Autodesk Inventor part; units mm, degrees
ref_plane "YZ Plane" through (0, 0, 0) normal (1, 0, 0) x (0, 1, 0)
ref_plane "XZ Plane" through (0, 0, 0) normal (0, 1, 0) x (-1, 0, 0)
ref_plane "XY Plane" through (0, 0, 0) normal (0, 0, 1) x (1, 0, 0)
sketch "Sketch1" plane through (0, 0, 0) normal (0, 1, 0) x (-1, 0, 0)
  line L0 (0, 0) -> (38.1, -25.4)
  line L1 (38.1, -25.4) -> (0, -25.4)
  line L2 (0, -25.4) -> (0, -57.5469)
  line L3 (0, -57.5469) -> (-28.575, -25.4)
  line L4 (-28.575, -25.4) -> (0, 0)
  dimension "d0" = 38.1
  dimension "d2" = 25.4
  dimension "d3" = 28.575
extrude "Extrusion1" add sketch "Sketch1" along normal blind 25.4
sketch "Sketch2" plane through (0, 25.4, 0) normal (0, 1, 0) x (1, 0, 0)
  line L0 (-38.1, 25.4) -> (0, 0)
  line L1 (-11.9592, 7.9728) -> (19.3376, 35.7921)
  line L2 (0, 0) -> (28.575, 25.4)
  line L3 (28.575, 25.4) -> (0, 57.5469)
  point P0 (0, 25.4)
  dimension "d6" = 5.08
extrude "Extrusion2" cut sketch "Sketch2" against normal blind 49.2125
sketch "Sketch3" plane through (19.3376, 0, -35.7921) normal (0.6643638, 0, 0.7474093) x (0.7474093, 0, -0.6643638)
  line L0 (-32.3668, 19.05) -> (-9.5068, 19.05)
  line L1 (-9.5068, 19.05) -> (-9.5068, 6.35)
  line L2 (-9.5068, 6.35) -> (-32.3668, 6.35)
  line L3 (-32.3668, 6.35) -> (-32.3668, 19.05)
  line L4 (0, 25.4) -> (0, 0)
  line L5 (-41.8736, 25.4) -> (0, 25.4)
  point P0 (-38.2321, 0)
  point P1 (-9.5068, 12.7)
  point P2 (0, 12.7)
  point P3 (-20.9368, 19.05)
  point P4 (-20.9368, 25.4)
  dimension "d9" = 12.7
  dimension "d10" = 22.86
extrude "Extrusion3" cut sketch "Sketch3" against normal blind 82.55
sketch "Sketch4" plane through (19.3376, 0, -35.7921) normal (0.6643638, 0, 0.7474093) x (0.7474093, 0, -0.6643638)
  point P0 (-38.2321, 0)
sketch "Sketch5" plane through (19.3376, 0, -35.7921) normal (0.6643638, 0, 0.7474093) x (0.7474093, 0, -0.6643638)
  line L0 (-9.5068, 6.35) -> (-9.5068, 19.05)
  line L1 (-9.5068, 15.24) -> (-6.9668, 15.24)
  line L2 (-6.9668, 15.24) -> (-6.9668, 10.16)
  line L3 (-6.9668, 10.16) -> (-9.5068, 10.16)
  line L4 (-9.5068, 10.16) -> (-9.5068, 15.24)
  point P0 (-38.2321, 0)
  point P1 (-6.9668, 12.7)
  point P2 (-9.5068, 12.7)
  dimension "d13" = 2.54
  dimension "d14" = 5.08
extrude "Extrusion4" cut sketch "Sketch5" against normal blind 36.5125
sketch "Sketch7" plane through (0, 0, -25.4) normal (0, 0, -1) x (-1, 0, 0)
  line L0 (0, 25.4) -> (38.1, 25.4)
  line L1 (38.1, 0) -> (38.1, 31.4433)
  line L2 (38.1, 31.4433) -> (13.5942, 73.8886)
  line L3 (0, 66.04) -> (0, 19.05)
  line L4 (13.5942, 73.8886) -> (0, 66.04)
  point P0 (0, 0)
extrude "Extrusion6" add sketch "Sketch7" against normal blind 20.6375
sketch "Sketch8" plane through (-38.1, 25.4, -4.7625) normal (0, -1, 0) x (1, 0, 0)
  line L0 (0, -20.6375) -> (26.1408, -3.2103)
  line L1 (26.1408, -3.2103) -> (38.1, -13.8407)
  line L2 (38.1, -13.8407) -> (38.1, 0)
  line L3 (0, 0) -> (38.1, 0)
  line L4 (0, -20.6375) -> (0, 0)
  point P0 (38.1, 4.7625)
extrude "Extrusion7" cut sketch "Sketch8" against normal blind 74.6125
sketch "Sketch9" plane through (0, 25.4, -25.4) normal (1, 0, 0) x (0, 0, -1)
  line L0 (0, 0) -> (-6.7968, 0)
  line L1 (-17.4272, -25.4) -> (-17.4272, 47.5446)
  line L2 (0, 0) -> (-17.4272, 0)
  line L3 (-17.4272, 0) -> (0, 48.4886)
  line L4 (0, 48.4886) -> (-17.4272, 48.4886)
  line L5 (-17.4272, 48.4886) -> (-17.4272, 0)
  point P0 (-25.4, -25.4)
extrude "Extrusion8" cut sketch "Sketch9" against normal blind 92.075
sketch "Sketch10" plane through (0, 25.4, 0) normal (0, 1, 0) x (1, 0, 0)
  line L0 (0, 25.4) -> (0, 18.6032)
  line L1 (0, 18.6032) -> (19.3376, 35.7921)
  line L2 (19.3376, 35.7921) -> (0, 57.5469)
  line L3 (0, 57.5469) -> (0, 25.4)
  line L4 (5.08, 51.054) -> (5.08, 24.93)
  line L5 (5.08, 24.93) -> (5.08, 23.1187)
  line L6 (5.08, 52.3795) -> (5.08, 51.054)
  point P0 (0, 0)
extrude "Extrusion9" add sketch "Sketch10" along normal blind 25.4
ref_plane "Work Plane1" through (0, -6.35, -128.016) normal (0, 0, -1) x (0, 1, 0)
sketch "Sketch11" plane through (0, -6.35, -128.016) normal (0, 0, -1) x (0, 1, 0)
  line L0 (57.15, 19.3376) -> (57.15, 0)
  line L1 (57.15, 0) -> (31.75, 19.3376)
  line L2 (57.15, 19.3376) -> (6.35, 19.3376)
  line L3 (31.75, 19.3376) -> (57.15, 19.3376)
  line L4 (57.15, 19.3376) -> (57.15, 0)
  point P0 (6.35, 0)
  dimension "d27" = 25.4
extrude "Extrusion10" cut sketch "Sketch11" against normal blind 209.55
sketch "Sketch12" plane through (0, 0, -57.5469) normal (-1, 0, 0) x (0, 0, 1)
  circle A0 centre (19.3199, 35.56) radius 1.778
  line L0 (6.4929, 66.04) -> (6.4929, 0)
  line L1 (0, 50.8) -> (32.1469, 50.8)
  point P0 (57.5469, 0)
  dimension "d30" = 3.556
  dimension "d31" = 12.827
  dimension "d32" = 15.24
extrude "Extrusion11" cut sketch "Sketch12" against normal blind 209.55
ref_plane "Work Plane2" through (2.54, 0, -57.5469) normal (-1, 0, 0) x (0, 0, 1)
sketch "Sketch13" plane through (2.54, 0, -57.5469) normal (-1, 0, 0) x (0, 0, 1)
  circle A0 centre (19.3199, 35.56) radius 1.778
  circle A1 centre (19.3199, 35.56) radius 3.81
  point P0 (57.5469, 0)
  dimension "d36" = 7.62
extrude "Extrusion12" cut sketch "Sketch13" against normal blind 209.55 contours A0 | A1
sketch "Sketch14" plane through (0, 0, -25.4) normal (0, 0, -1) x (-1, 0, 0)
  circle A0 centre (25.4, 25.4) radius 1.778
  line L0 (38.1, 0) -> (38.1, 31.4433)
  line L1 (0, 0) -> (38.1, 0)
  dimension "d39" = 3.556
  dimension "d40" = 12.7
  dimension "d41" = 25.4
extrude "Extrusion13" cut sketch "Sketch14" against normal blind 115.8875
ref_plane "Work Plane3" through (0, 0, -22.86) normal (0, 0, -1) x (-1, 0, 0)
sketch "Sketch15" plane through (0, 0, -22.86) normal (0, 0, -1) x (-1, 0, 0)
  circle A0 centre (25.4, 25.4) radius 1.778
  circle A1 centre (25.4, 25.4) radius 3.81
  point P0 (0, 0)
  dimension "d45" = 7.62
extrude "Extrusion14" cut sketch "Sketch15" against normal blind 115.8875
sketch "Sketch16" plane through (0, 0, 0) normal (0, -1, 0) x (1, 0, 0)
  circle A0 centre (-11.9592, -15.5928) radius 1.778
  point P0 (0, 0)
extrude "Extrusion15" cut sketch "Sketch16" against normal blind 15.24
sketch "Sketch17" plane through (-11.9592, 0, -7.9728) normal (0.6643638, 0, 0.7474093) x (0.7474093, 0, -0.6643638)
  circle A0 centre (6.9668, 12.8573) radius 0.889
  circle A1 centre (34.9068, 12.8573) radius 0.889
  line L0 (32.3668, 6.35) -> (9.5068, 6.35)
  point P0 (3.6416, 0)
  point P1 (20.9368, 6.35)
  dimension "d50" = 27.94
  dimension "d51" = 1.778
  dimension "d52" = 1.778
  dimension "d53" = 13.97
extrude "Extrusion16" cut sketch "Sketch17" against normal blind 3.81 contours A0
sketch "Sketch19" plane through (0, 0, 0) normal (0, -1, 0) x (1, 0, 0)
  line L0 (-16.51, -25.4) -> (-14.7303, -25.4)
  line L1 (-16.51, -25.4) -> (-23.1531, -15.4354)
  line L2 (-29.21, -19.4733) -> (-21.59, -14.3933)
  line L3 (-11.43, -25.4) -> (-17.5429, -11.6953)
  line L4 (-11.9592, -7.9728) -> (-26.2667, -17.5112)
  line L5 (0, -25.4) -> (-38.1, -25.4)
  point P0 (0, 0)
extrude "Extrusion18" cut sketch "Sketch19" against normal blind 7.62
chamfer "Chamfer1" distance 1.5875 angle 45 1 edges at (-17.5429, 3.81, -11.6953)
properties part number "Thumb Base2"
Geometry check sheet. Reference: the model listing, model coordinates, mm. A direction names the side the tool comes from. Round coordinates to 2 decimals unless told otherwise and drop trailing zeros. Write each loop counter-clockwise with the first axis right and the second up, starting at its lowest first coordinate (ties: lowest second). Pieces come first, ordered by that corner, then holes.
Item 1: Material ranges on line 1 along Y through (x, z) = (-25.4, -19.75); line 2 along Y through (x, z) = (-27.5, -19); line 3 along Z through (x, y) = (6, 35.56), recorded low to high.
Determined:
line 1: y = 0 to 21.59, 29.21 to 53.44
line 2: y = 0 to 22.22, 28.58 to 49.8
line 3: z = -50.8 to -42.04, -34.42 to -23.94
Item 2: Section check C-C (z = -48). Record the boundary of the cut face in (x, y).
Determined:
outline: (0, 0) - (8.49, 0) - (8.49, 39.65) - (0, 50.8) - close
Item 3: Access from +Z, -Z, +X, -X, +Y, -Y to the whole of each face (thin tool, end or side, straight path). Record for faces 5 (the face through (-21.594, 25.568, -19.613)), 6 (the face through (0, 57, -23)), 7 (the face through (-12, 15.24, -16)), 8 (the face through (7.164, 12.736, -39.001)).
Determined:
face 5: +Z
face 6: +Z, -Z, +X, +Y
face 7: -Y
face 8: +Z, -X
Item 4: Section check D-D (y = 65). Record the boundary of the cut face in (x, z), plus the area to 3 significant figures.
Determined:
outline: (-18.73, -25.4) - (0, -25.4) - (0, -22.21) - (-18.73, -22.21) - close
area: 59.8 mm2
Item 5: Go/stop test with flat-tipped pins: pin 1 Ø12 at (y, z) = (35.56, -38.227) entering from -X; pin 2 Ø3 at (x, z) = (-17.5, -16) entering from -Y; pin 3 Ø3 at (x, y) = (-7, 3.5) entering from -Z; pin 4 Ø13.5 at (x, z) = (-2, -25.5) entering from -Y. Record where each tip stops, or that it passes through.
Determined:
pin 1: stops at x = 0
pin 2: stops at y = 7.62
pin 3: stops at z = -25.4
pin 4: stops at y = 0
Item 6: Mould release check, pull along X, two halves, no side actions. Record for faces 1 (the face through (-24.847, 19.835, -16.564)), 2 (the face through (-24, 24, -22.86)), 3 (the face through (-9.723, 12.611, -19.767)), 4 (the face through (-18, 7.62, -18)): +X half, -X half, draft (parallel to the pull), parting line (faces both ways), or undercut.
Determined:
face 1: -X half
face 2: undercut
face 3: +X half
face 4: undercut
Item 7: Section check B-B (x = -25.4). Record the boundary of the cut face in (y, z), plus the area to 3 significant figures.
Determined:
outline: (0, -25.4) - (23.62, -25.4) - (23.62, -22.86) - (21.59, -22.86) - (21.59, -16.93) - (0, -16.93) - close; (27.18, -25.4) - (53.44, -25.4) - (53.44, -18.05) - (50.33, -16.93) - (29.21, -16.93) - (29.21, -22.86) - (27.18, -22.86) - close
area: 397 mm2
Item 8: Section check A-A (y = 35.56). Record the boundary of the cut face in (x, z) (3 decimals), plus the area to 3 significant figures.
Determined:
outline: (-35.723, -25.4) - (0, -25.4) - (0, -36.449) - (2.54, -36.449) - (2.54, -34.417) - (11.603, -34.417) - (11.603, -28.917) - (0, -18.603) - (-7.851, -11.624) - (-17.437, -11.624) - (-35.723, -23.815) - close; (0, -57.547) - (11.603, -44.494) - (11.603, -42.037) - (2.54, -42.037) - (2.54, -40.005) - (0, -40.005) - close
area: 591 mm2
